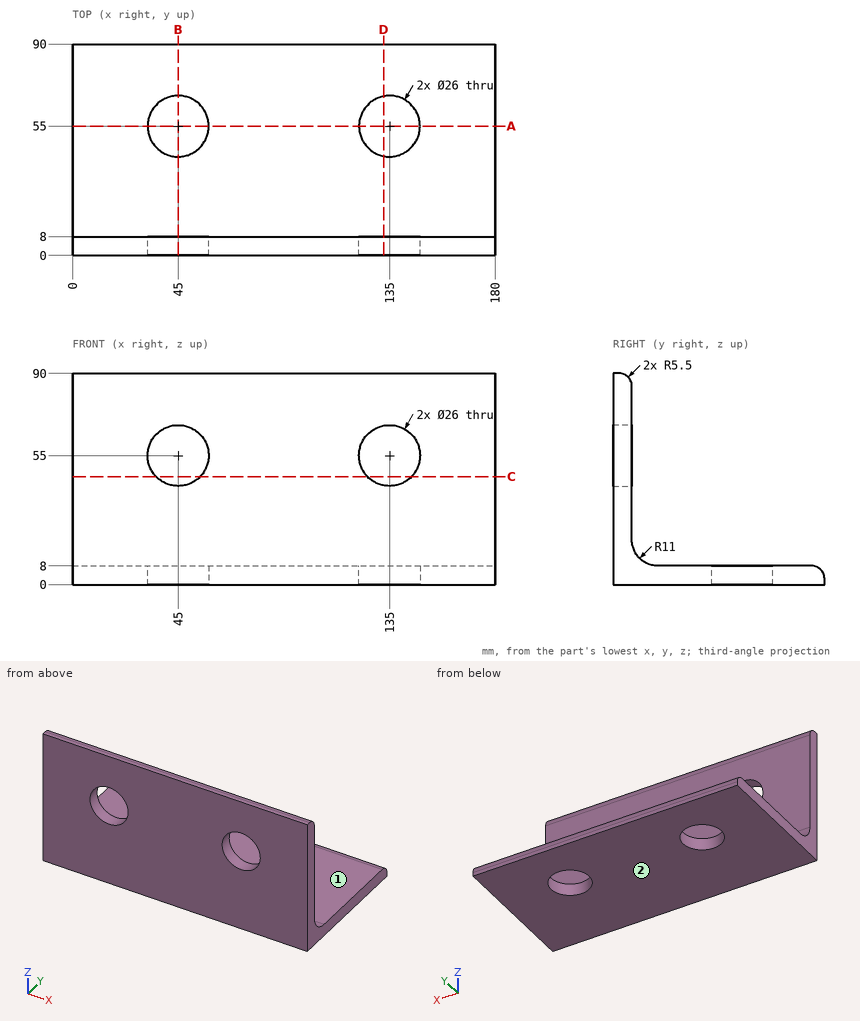
Input: dimensioned drawing with shaded views. Units: mm. Origin: part minimum x, y, z. A direction names the side the tool comes from. Coordinates: 2 decimals unless noted, no trailing zeros. Order: outer loops, then holes, each group sorted by start corner. A loop starts at its lowest first (then second) coordinate and runs counter-clockwise, first axis right, second up. Notation, with made-up numbers: M 69.5,57 L 113.5,57 A14 ccw 113.5,80 Z; hole C 11.5,77 d3. An arc over 180 degrees is marked long. Write each question's results on one line, items separated by ' | '. Start each with the question number.
Item 1: First-contact query: pin 1 Ø1 at (x, y) = (66, 17.5) entering from -Z; pin 2 Ø8 at (x, z) = (110, 35) entering from +Y; pin 3 Ø6 at (x, y) = (75.5, 13) entering from +Z; pin 4 Ø19.5 at (x, y) = (62, 50) entering from +Z. Flat tips, straight axial feed; report the tip coordinate or a pass-through.
Item 2: Line query: probe 1 along X at (y, z) = (1.5, 55); probe 2 along Z at (x, y) = (135, 2); probe 3 along Y at (x, z) = (127, 26). Output: solid intervals per line, ascending.
Item 3: Cut plane C-C (z = 46). Return loops of the section in (x, y), and give its area (3 significant figures).
Item 4: Cut plane B-B (x = 45). Return loops of the section in (y, z).
Item 5: Set-up query: the marked faces 1 and 2. Return all of +Z, -Z, +X, -X, +Y, -Y with unobstructed straight access to the full face (end or side cutting, diameter ignored); none if empty.
Item 6: Cut plane A-A (y = 55). Return loops of the section in (x, z).
Item 7: Cut plane D-D (x = 132.5). Return loops of the section in (y, z), and give its area (3 significant figures).
Checked values:
1) pin 1: stops at z = 0 | pin 2: stops at y = 8 | pin 3: stops at z = 12.68 | pin 4: stops at z = 8
2) probe 1: x = 0 to 32, 58 to 122, 148 to 180 | probe 2: z = 0 to 42, 68 to 90 | probe 3: y = 0 to 8
3) outline: M 0,0 L 35.62,0 L 35.62,8 L 0,8 Z; M 54.38,0 L 125.62,0 L 125.62,8 L 54.38,8 Z; M 144.38,0 L 180,0 L 180,8 L 144.38,8 Z | area: 1,140 mm2
4) outline: M 0,0 L 42,0 L 42,8 L 19,8 A11 cw 8,19 L 8,42 L 0,42 Z; M 0,68 L 8,68 L 8,84.5 A5.5 ccw 2.5,90 L 0,90 Z; M 68,0 L 90,0 L 90,2.5 A5.5 ccw 84.5,8 L 68,8 Z
5) face 1: +Z, +X, -X, +Y | face 2: -Z, +X, -X, +Y, -Y
6) outline: M 0,0 L 32,0 L 32,8 L 0,8 Z; M 58,0 L 122,0 L 122,8 L 58,8 Z; M 148,0 L 180,0 L 180,8 L 148,8 Z
7) outline: M 0,0 L 42.24,0 L 42.24,8 L 19,8 A11 cw 8,19 L 8,42.24 L 0,42.24 Z; M 0,67.76 L 8,67.76 L 8,84.5 A5.5 ccw 2.5,90 L 0,90 Z; M 67.76,0 L 90,0 L 90,2.5 A5.5 ccw 84.5,8 L 67.76,8 Z | area: 981 mm2
